Build history of the part. All positions in model axes, mm. A direction names the side the tool comes from. Coordinates: 2 decimals unless noted, no trailing zeros. Order: outer loops, then holes, each group sorted by start corner. A loop starts at its lowest first (then second) coordinate and runs counter-clockwise, first axis right, second up. Notation, with made-up numbers: (53, 6.25) - (106, 6.25) arc R19 ccw to (106, 39.25) - close; hole circle Ø1 at (37, 61). An arc over 180 degrees is marked (long way). Write each question's results on one line, items separated by ' | '. Start each with the question number.
from build123d import *

# Parameters (mm, degrees)
SKETCH1_W           = 15
SKETCH1_H           = 5
BOSS_EXTRUDE1_DEPTH = 5
CUT_EXTRUDE1_DEPTH  = 5
SKETCH3_W           = 5
SKETCH3_H           = 2.306580292
BOSS_EXTRUDE2_DEPTH = 5
BOSS_EXTRUDE3_DEPTH = 5


with BuildPart() as part:
    # Sketch1 → Boss-Extrude1 (new body)
    with BuildSketch(Plane(origin=(0, 0, 0), x_dir=(1, 0, 0), z_dir=(0, 1, 0))):
        with Locations((7.5, 2.5)):
            Rectangle(SKETCH1_W, SKETCH1_H)
    extrude(amount=BOSS_EXTRUDE1_DEPTH)

    # Sketch2 → Cut-Extrude1 (cut)
    with BuildSketch(Plane.XY):
        Polygon((3, 5), (12, 5), (13.120394862, 2.991339911), (2.986234937, 2.991339911), (2.986234937, 5), align=None)
    extrude(amount=-CUT_EXTRUDE1_DEPTH, mode=Mode.SUBTRACT)

    # Sketch3 → Boss-Extrude2 (add)
    with BuildSketch(Plane.ZY):
        with Locations((-2.5, 1.153290146)):
            Rectangle(SKETCH3_W, SKETCH3_H)
    extrude(amount=BOSS_EXTRUDE2_DEPTH)

    # Sketch7 → Boss-Extrude3 (add)
    with BuildSketch(Plane.XY):
        Polygon((-5, 0), (-13.001867805, 0), (-5, 2.306580292), align=None)
    extrude(amount=-BOSS_EXTRUDE3_DEPTH)

    # Cut-Loft1: read off the stored shape, not the designer's step
    # Cut-Loft1: loft between two sections, ruled curve by curve
    cut_loft1_from = [
        Edge.make_bspline([(10.775857545, 0, -3.733497041), (10.684223664, 0, -3.733497041), (10.580567417, 0, -3.722354361), (10.355367989, 0, -3.656671194), (10.233384966, 0, -3.601544251), (9.998802229, 0, -3.425607198), (9.886786943, 0, -3.303547063), (9.724445949, 0, -2.999157699), (9.676250966, 0, -2.817158224), (9.676250966, 0, -2.450622698), (9.724445949, 0, -2.268623224), (9.886786943, 0, -1.964233859), (9.998802229, 0, -1.842173724), (10.233384966, 0, -1.666236672), (10.355367989, 0, -1.611109728), (10.580567417, 0, -1.545426562), (10.684223664, 0, -1.534283882), (10.867491427, 0, -1.534283882), (10.971147674, 0, -1.545426562), (11.196347101, 0, -1.611109728), (11.318330124, 0, -1.666236672), (11.552912861, 0, -1.842173724), (11.664928148, 0, -1.964233859), (11.827269142, 0, -2.268623224), (11.875464125, 0, -2.450622698), (11.875464125, 0, -2.817158224), (11.827269142, 0, -2.999157699), (11.664928148, 0, -3.303547063), (11.552912861, 0, -3.425607198), (11.318330124, 0, -3.601544251), (11.196347101, 0, -3.656671194), (10.971147674, 0, -3.722354361), (10.867491427, 0, -3.733497041), (10.775857545, 0, -3.733497041)], [0, 0, 0, 0, 0.0625, 0.0625, 0.125, 0.125, 0.1875, 0.1875, 0.25, 0.25, 0.3125, 0.3125, 0.375, 0.375, 0.4375, 0.4375, 0.5, 0.5, 0.5625, 0.5625, 0.625, 0.625, 0.6875, 0.6875, 0.75, 0.75, 0.8125, 0.8125, 0.875, 0.875, 0.9375, 0.9375, 1, 1, 1, 1], 3),
    ]
    cut_loft1_to = [
        Edge.make_bspline([(15, 1.571629768, -3.022785324), (15, 1.59774719, -3.110618396), (15, 1.637971718, -3.206799289), (15, 1.765116639, -3.403936879), (15, 1.852724527, -3.505148024), (15, 2.088224624, -3.67985524), (15, 2.237148437, -3.752434842), (15, 2.575182586, -3.821285391), (15, 2.763369546, -3.815607976), (15, 3.114701834, -3.71113829), (15, 3.275415798, -3.613068993), (15, 3.520909325, -3.370704781), (15, 3.60598011, -3.228546199), (15, 3.70775901, -2.953548085), (15, 3.725831875, -2.820912459), (15, 3.724604446, -2.586332933), (15, 3.705740921, -2.483800283), (15, 3.653506078, -2.308134139), (15, 3.61328155, -2.211953246), (15, 3.486136629, -2.014815656), (15, 3.398528741, -1.913604511), (15, 3.163028644, -1.738897295), (15, 3.014104831, -1.666317693), (15, 2.676070682, -1.597467144), (15, 2.487883722, -1.603144559), (15, 2.136551433, -1.707614245), (15, 1.97583747, -1.805683542), (15, 1.730343943, -2.048047754), (15, 1.645273158, -2.190206336), (15, 1.543494258, -2.46520445), (15, 1.525421393, -2.597840076), (15, 1.526648822, -2.832419602), (15, 1.545512347, -2.934952252), (15, 1.571629768, -3.022785324)], [0, 0, 0, 0, 0.0625, 0.0625, 0.125, 0.125, 0.1875, 0.1875, 0.25, 0.25, 0.3125, 0.3125, 0.375, 0.375, 0.4375, 0.4375, 0.5, 0.5, 0.5625, 0.5625, 0.625, 0.625, 0.6875, 0.6875, 0.75, 0.75, 0.8125, 0.8125, 0.875, 0.875, 0.9375, 0.9375, 1, 1, 1, 1], 3),
    ]
    cut_loft1 = Solid(Shell([*[Face.make_surface_from_curves(cut_loft1_from[k], cut_loft1_to[k]) for k in range(1)], Face(Wire(cut_loft1_from)), Face(Wire(cut_loft1_to))]))
    add(cut_loft1, mode=Mode.SUBTRACT)


solid = part.part
Item 1: Slice it at C-C (x = -2.75). Write the cut outline in (y, z).
Item 2: Which spindle directions (+Z, -Z, +X, -X, +Y, -Y) get a long thin tool onto all of the face, cutting with end or side? Do faces 5 (the flat face through (12.55, 4.01, -2.46)), 6 (the flat face through (0, 4, -2)), 7 (the flat face through (4, 2, -5)). Say none if no direction does.
Item 3: Slice it at B-B (y = 4.55). Write the cut outline in (x, z), then the cut area to 3 significant figures.
Item 4: Pull direction X, two halves, no side cores. Call faces 1 (the flat face through (4, 2, 0)), 2 (the flat face through (2.986, 4, -2)), 3 (the flat face through (15, 1, -2)), 4 (the flat face through (-9.057, 1.137, -2.465)): released by +X, released by -X, zero draft, split by the parting line, or undercut.
Item 5: Probe probe 1 along Y at (x, z) = (-2.25, -0.75); probe 2 along X at (y, z) = (4.25, -0.45); probe 3 along Y at (x, z) = (6.75, -2.7). List the from-to ranges inside material, lowest first.
Item 6: Slice it at A-A (z = -0.35). Write the cut outline in (x, y).
Item 7: Slice it at D-D (x = 7.5). Write the cut outline in (y, z).
Item 8: Flat gauge pins, fed straight in: P1, Ø2, axis at x = -3, y = 4, coming from the -Z side; P2, Ø1.5, axis at x = -1.5, z = -2, coming from the +Y side; P3, Ø2, axis at y = 3.5, z = -2.5, coming from the -X side; P4, Ø3, axis at x = -7, y = 2.5, coming from the -Z side. Where does each tip first touch, or does it go through?
Resolved:
1) outline: (0, -5) - (2.31, -5) - (2.31, 0) - (0, 0) - close
2) face 5: +Z, -Z | face 6: +Z, -Z, -X, +Y | face 7: -Z, +X, -X, +Y, -Y
3) outline: (0, -5) - (2.99, -5) - (2.99, 0) - (0, 0) - close; (12.25, -5) - (15, -5) - (15, 0) - (12.25, 0) - close | area: 28.7 mm^2
4) face 1: zero draft | face 2: undercut | face 3: released by +X | face 4: released by -X
5) probe 1: 0 to 2.31 | probe 2: 0 to 2.99, 12.42 to 15 | probe 3: 0 to 2.99
6) outline: (-13, 0) - (15, 0) - (15, 5) - (12, 5) - (13.12, 2.99) - (2.99, 2.99) - (2.99, 5) - (0, 5) - (0, 2.31) - (-5, 2.31) - close
7) outline: (0, -5) - (2.99, -5) - (2.99, 0) - (0, 0) - close
8) P1: through | P2: y = 2.31 | P3: x = 0 | P4: z = -5
